Verification items for the finished model (mm, model axes). A direction names the side the tool comes from. Round coordinates to 2 decimals unless told otherwise and drop trailing zeros. Write each loop counter-clockwise with the first axis right and the second up, starting at its lowest first coordinate (ties: lowest second). Pieces come first, ordered by that corner, then holes. Notation, with made-up numbers: M 73.5,60.25 L 119.5,60.25 A23 cw 119.5,89.25 Z; hole C 4.5,25 d9. An arc over 180 degrees is marked long. One line per item, written item: value. Start each with the question number.
Item 1: Tool access check on faces 4 (the face through (5, 6, -5)), 5 (the face through (40, 3, -2)), 6 (the face through (57, 3, -9)), 7 (the face through (5.07, 2.155, -5.921)), 8 (the face through (65, 5, -6)). Record the directions out of +Z, -Z, +X, -X, +Y, -Y that give a thin tool (end or side, any length) a straight path to the whole face; none if there is none.
Item 2: Section check C-C, the plane x = 58.5. Record the cut outline in (y, z) (3 decimals).
Item 3: Section check A-A, the plane x = 14. Record the cut outline in (y, z).
Item 4: Section check B-B, the plane x = 30. Record the cut outline in (y, z).
Item 5: Draft check along Z on faces 1 (the face through (23, 3, -9)), 2 (the face through (15.24, 3.27, -5.16)), 3 (the face through (23, 3, -1)). Enter one of: +Z half, -Z half, draft (parallel to the pull), parting line (faces both ways), or undercut.
Item 6: Gauge pin test, flat ends, axial feed: pin 1 (4 mm diameter, centred on x = 14, z = -5, fed in from -Y); pin 2 (2 mm diameter, centred on x = 66, z = -5, fed in from -Y); pin 3 (1 mm diameter, centred on x = 26.5, y = 1, fed in from +Z); pin 4 (1.5 mm diameter, centred on x = 20.5, y = 3, fed in from +Z). Record the tip position at first contact, or that the pin passes through.
Item 7: Thickness scan on probe 1 along Y at (x, z) = (7, -5); probe 2 along Z at (x, y) = (66, 2.35); probe 3 along X at (y, z) = (3.45, -5.5). Record the ranges inside material, lowest first. Write a range as from..to.
from build123d import *

# Parameters (mm, degrees)
SKETCH1_W                                 = 80
SKETCH1_H                                 = 10
BOSS_EXTRUDE1_DEPTH                       = 6
SKETCH2_W                                 = 6
SKETCH2_H                                 = 10
CUT_EXTRUDE1_DEPTH                        = 1
TAP_DRILL_FOR_M3X0_5_TAP1_D               = 2.5
TAP_DRILL_FOR_M3X0_5_TAP1_DEPTH           = 10
TAP_DRILL_FOR_M3X0_5_TAP1_TIP             = 0.751075774
TAP_DRILL_FOR_M3X0_5_TAP1_ON_FACE_2_D     = 2.5
TAP_DRILL_FOR_M3X0_5_TAP1_ON_FACE_2_DEPTH = 10
TAP_DRILL_FOR_M3X0_5_TAP1_ON_FACE_2_TIP   = 0.751075774
TAP_DRILL_FOR_M3X0_5_TAP1_ON_FACE_3_D     = 2.5
TAP_DRILL_FOR_M3X0_5_TAP1_ON_FACE_3_DEPTH = 10
TAP_DRILL_FOR_M3X0_5_TAP1_ON_FACE_3_TIP   = 0.751075774
CHAMFER1_SIZE                             = 1.5
CUT_EXTRUDE2_REACH                        = 82.846
FILLET1_R                                 = 5


with BuildPart() as part:
    # Sketch1 → Boss-Extrude1 (new body)
    with BuildSketch(Plane(origin=(0, 0, 0), x_dir=(1, 0, 0), z_dir=(0, 1, 0))):
        with Locations((40, 5)):
            Rectangle(SKETCH1_W, SKETCH1_H)
    extrude(amount=BOSS_EXTRUDE1_DEPTH)

    # Sketch2 → Cut-Extrude1 (cut)
    with BuildSketch(Plane(origin=(0, 6, 0), x_dir=(1, 0, 0), z_dir=(0, 1, 0))):
        with Locations((14, 5)):
            Rectangle(SKETCH2_W, SKETCH2_H)
        with Locations((66, 5)):
            Rectangle(SKETCH2_W, SKETCH2_H)
    extrude(amount=-CUT_EXTRUDE1_DEPTH, mode=Mode.SUBTRACT)

    # Tap Drill for M3x0.5 Tap1
    with Locations(Plane(origin=(80, 3, -5), x_dir=(0, 0, 1), z_dir=(1, 0, 0))):
        with Locations((0, 0)):
            Hole(TAP_DRILL_FOR_M3X0_5_TAP1_D / 2, depth=TAP_DRILL_FOR_M3X0_5_TAP1_DEPTH)
            with Locations((0, 0, -(TAP_DRILL_FOR_M3X0_5_TAP1_DEPTH + TAP_DRILL_FOR_M3X0_5_TAP1_TIP / 2))):  # 118° drill point
                Cone(0, TAP_DRILL_FOR_M3X0_5_TAP1_D / 2, TAP_DRILL_FOR_M3X0_5_TAP1_TIP, mode=Mode.SUBTRACT)

    # Tap Drill for M3x0.5 Tap1 on face 2
    with Locations(Plane(origin=(66, 0, -5), x_dir=(0, 0, -1), z_dir=(0, -1, 0))):
        with Locations((0, 0), (0, -52)):
            Hole(TAP_DRILL_FOR_M3X0_5_TAP1_ON_FACE_2_D / 2, depth=TAP_DRILL_FOR_M3X0_5_TAP1_ON_FACE_2_DEPTH)
            with Locations((0, 0, -(TAP_DRILL_FOR_M3X0_5_TAP1_ON_FACE_2_DEPTH + TAP_DRILL_FOR_M3X0_5_TAP1_ON_FACE_2_TIP / 2))):  # 118° drill point
                Cone(0, TAP_DRILL_FOR_M3X0_5_TAP1_ON_FACE_2_D / 2, TAP_DRILL_FOR_M3X0_5_TAP1_ON_FACE_2_TIP, mode=Mode.SUBTRACT)

    # Tap Drill for M3x0.5 Tap1 on face 3
    with Locations(Plane(origin=(0, 3, -5), x_dir=(0, 0, -1), z_dir=(-1, 0, 0))):
        with Locations((0, 0)):
            Hole(TAP_DRILL_FOR_M3X0_5_TAP1_ON_FACE_3_D / 2, depth=TAP_DRILL_FOR_M3X0_5_TAP1_ON_FACE_3_DEPTH)
            with Locations((0, 0, -(TAP_DRILL_FOR_M3X0_5_TAP1_ON_FACE_3_DEPTH + TAP_DRILL_FOR_M3X0_5_TAP1_ON_FACE_3_TIP / 2))):  # 118° drill point
                Cone(0, TAP_DRILL_FOR_M3X0_5_TAP1_ON_FACE_3_D / 2, TAP_DRILL_FOR_M3X0_5_TAP1_ON_FACE_3_TIP, mode=Mode.SUBTRACT)

    # Chamfer1
    chamfer1_edges = [part.edges().sort_by_distance(p)[0] for p in [
        (14, 0, -6.25),
        (66, 0, -6.25),
    ]]
    chamfer(chamfer1_edges, length=CHAMFER1_SIZE)

    # Sketch6 → Cut-Extrude2 (cut, up to next)
    with BuildSketch(Plane(origin=(0, 6, 0), x_dir=(1, 0, 0), z_dir=(0, 1, 0)), mode=Mode.PRIVATE) as cut_extrude2_sk1:
        Polygon((19, 10), (27, 8), (53, 8), (61, 10), align=None)
    cut_extrude2_tool1 = extrude(cut_extrude2_sk1.sketch, amount=-CUT_EXTRUDE2_REACH, mode=Mode.PRIVATE) & part.part
    # Sketch6 → Cut-Extrude2 (cut, up to next)
    with BuildSketch(Plane(origin=(0, 6, 0), x_dir=(1, 0, 0), z_dir=(0, 1, 0)), mode=Mode.PRIVATE) as cut_extrude2_sk2:
        Polygon((19, 0), (27, 2), (53, 2), (61, 0), align=None)
    cut_extrude2_tool2 = extrude(cut_extrude2_sk2.sketch, amount=-CUT_EXTRUDE2_REACH, mode=Mode.PRIVATE) & part.part
    add(cut_extrude2_tool1.solids().sort_by_distance((40, 6, -9.078431))[0], mode=Mode.SUBTRACT)
    add(cut_extrude2_tool2.solids().sort_by_distance((40, 6, -0.921569))[0], mode=Mode.SUBTRACT)

    # Fillet1
    fillet1_edges = [part.edges().sort_by_distance(p)[0] for p in [
        (19, 3, -10),
        (61, 3, -10),
        (53, 3, -8),
        (27, 3, -8),
        (61, 3, 0),
        (19, 3, 0),
        (27, 3, -2),
        (53, 3, -2),
    ]]
    fillet(fillet1_edges, radius=FILLET1_R)


solid = part.part
Response values:
1. face 4: +Z, -Z, +X, -X, +Y
1. face 5: +Z, +Y, -Y
1. face 6: -Z, +Y, -Y
1. face 7: -X
1. face 8: +Z, -Z, +Y
2. outline: M 0,-9.375 L 6,-9.375 L 6,-0.625 L 0,-0.625 Z
3. outline: M 0,-10 L 5,-10 L 5,-6.25 L 1.5,-6.25 L 0,-7.75 Z; M 0,-2.25 L 1.5,-3.75 L 5,-3.75 L 5,0 L 0,0 Z
4. outline: M 0,-8 L 6,-8 L 6,-2 L 0,-2 Z
5. face 1: -Z half
5. face 2: undercut
5. face 3: +Z half
6. pin 1: stops at y = 0.75
6. pin 2: passes through
6. pin 3: stops at z = -1.75
6. pin 4: stops at z = -0.19
7. probe 1: y = 0..1.75, 4.25..6
7. probe 2: z = -10..-6.25, -3.75..0
7. probe 3: x = 10.35..12.85, 15.15..64.85, 67.15..69.65
